```python
from build123d import *

# Parameters (mm, degrees)
BOSS_EXTRUDE1_DEPTH = 3
SKETCH2_R           = 1.75
CUT_EXTRUDE1_DEPTH  = 121.037494142
FILLET2_R           = 5


with BuildPart() as part:
    # Sketch1 → Boss-Extrude1 (new body)
    with BuildSketch(Plane(origin=(0, 0, 0), x_dir=(1, 0, 0), z_dir=(0, 1, 0))):
        Polygon((0, 0), (-84.852813742, 84.852813742), (-54.852813742, 84.852813742), (0, 30), align=None)
    extrude(amount=BOSS_EXTRUDE1_DEPTH)

    # Sketch2 → Cut-Extrude1 (cut, through all)
    with BuildSketch(Plane(origin=(0, 3, 0), x_dir=(1, 0, 0), z_dir=(0, 1, 0))):
        with Locations(Location((-69.852813742, 74.852813742, 0), (0, 0, 270))):
            Circle(SKETCH2_R)
        with Locations(Location((-49.852813742, 74.852813742, 0), (0, 0, 270))):
            Circle(SKETCH2_R)
        with Locations(Location((-10, 15, 0), (0, 0, 270))):
            Circle(SKETCH2_R)
        with Locations(Location((-10, 35, 0), (0, 0, 270))):
            Circle(SKETCH2_R)
    extrude(amount=-CUT_EXTRUDE1_DEPTH, mode=Mode.SUBTRACT)

    # Fillet2
    fillet2_edges = [part.edges().sort_by_distance(p)[0] for p in [
        (0, 1.5, 0),
        (-84.852813742, 1.5, -84.852813742),
        (-54.852813742, 1.5, -84.852813742),
        (0, 1.5, -30),
    ]]
    fillet(fillet2_edges, radius=FILLET2_R)


solid = part.part
```
Check sheet for the modelled part. Datum: model origin and axes. Units: mm. Round coordinates to 2 decimals unless told otherwise and drop trailing zeros. Write each loop counter-clockwise with the first axis right and the second up, starting at its lowest first coordinate (ties: lowest second). Pieces come first, ordered by that corner, then holes. Notation, with made-up numbers: M 85,24 L 100,24 A25 ccw 100,50 Z; hole C 25,-28 d3. An arc over 180 degrees is marked long. Write item = value, one per line. Start each with the question number.
1. Release check for a two-part mould opening along Z. For faces 1 (the flat face through (-42, 1, -42)), 2 (the cylindrical face through (-8.82, 1.52, -36.29)), 3 (the flat face through (-36, 0, -52)) record: pulls with the +Z half, pulls with the -Z half, needs draft (parallel to the pull), parting line crosses it, or undercut.
2. Scan lines: line 1 (Z direction, x = -9.5, y = 2.2); line 2 (Z direction, x = -51, y = 0.6); line 3 (X direction, y = 0.8, z = -75.5). Record each from-to range of solid material in increasing order. Write a range as [from, to].
3. Section check A-A, the plane x = -10. Record the cut outline in (y, z), then the cut area to 3 significant figures.
4. Section check C-C, the plane y = 2.45. Record the cut outline in (x, z), then the cut area to 3 significant figures.
5. Section check D-D, the plane z = -15. Record the cut outline in (x, y), then the cut area to 3 significant figures.
6. Section check B-B, the plane z = -35. Record the cut outline in (x, y), then the cut area to 3 significant figures.
Results found:
q1.face_1 = pulls with the +Z half
q1.face_2 = undercut
q1.face_3 = needs draft
q2.line_1 = [-39.5, -36.68], [-33.32, -16.68], [-13.32, -9.5]
q2.line_2 = [-81, -76.17], [-73.53, -51]
q2.line_3 = [-75.5, -71.48], [-68.23, -51.48], [-48.23, -45.5]
q3.outline = M 0,-40 L 3,-40 L 3,-36.75 L 0,-36.75 Z; M 0,-33.25 L 3,-33.25 L 3,-16.75 L 0,-16.75 Z; M 0,-13.25 L 3,-13.25 L 3,-10 L 0,-10 Z
q3.area = 69.0 mm^2
q4.outline = M -76.32,-76.32 A5 ccw -72.78,-84.85 L -56.92,-84.85 A5 ccw -53.39,-83.39 L -1.46,-31.46 A5 ccw 0,-27.93 L 0,-12.07 A5 ccw -8.54,-8.54 Z; hole C -69.85,-74.85 d3.5; hole C -49.85,-74.85 d3.5; hole C -10,-35 d3.5; hole C -10,-15 d3.5
q4.area = 1,990 mm^2
q5.outline = M -15,0 L -11.75,0 L -11.75,3 L -15,3 Z; M -8.25,0 L 0,0 L 0,3 L -8.25,3 Z
q5.area = 34.5 mm^2
q6.outline = M -35,0 L -11.75,0 L -11.75,3 L -35,3 Z; M -8.25,0 L -5,0 L -5,3 L -8.25,3 Z
q6.area = 79.5 mm^2
